from build123d import *

# Parameters (mm, degrees)
CYLINDER011_R     = 2.2
CYLINDER011_DEPTH = 10
CYLINDER012_R     = 2.2
CYLINDER012_DEPTH = 10
PAD015_DEPTH      = 6
CYLINDER013_R     = 4.5
CYLINDER013_DEPTH = 8


with BuildPart() as obj1:
    # Cylinder011 → Cylinder011 (new body)
    with BuildSketch(Plane(origin=(5, 0, -2), x_dir=(1, 0, 0), z_dir=(0, 0, 1))):
        Circle(CYLINDER011_R)
    extrude(amount=CYLINDER011_DEPTH)


with BuildPart() as double_hole_fusion:
    # Cylinder012 → Cylinder012 (new body)
    with BuildSketch(Plane(origin=(-5, 0, -2), x_dir=(1, 0, 0), z_dir=(0, 0, 1))):
        Circle(CYLINDER012_R)
    extrude(amount=CYLINDER012_DEPTH)

    # Fusion010: union obj1
    add(obj1.part)


with BuildPart() as body016:
    # Sketch016 → Pad015 (new body)
    with BuildSketch(Plane.XY):
        with BuildLine():
            Line((-5, 8), (5, 8))
            ThreePointArc((5, -8), (13, 0), (5, 8))
            Line((-5, -8), (5, -8))
            ThreePointArc((-5, 8), (-13, 0), (-5, -8))
        make_face()
    extrude(amount=PAD015_DEPTH)


with BuildPart() as simple_idle_linkage_cut:
    # Cylinder013 → Cylinder013 (new body)
    with BuildSketch(Plane(origin=(5, 0, 0), x_dir=(1, 0, 0), z_dir=(0, 0, 1))):
        Circle(CYLINDER013_R)
    extrude(amount=CYLINDER013_DEPTH)

    # Fusion011: union Body016
    add(body016.part)

    # Cut004: cut double hole fusion
    add(double_hole_fusion.part, mode=Mode.SUBTRACT)


solid = simple_idle_linkage_cut.part
Geometry: final body of the model. Coordinates: model frame, mm. Round coordinates to 2 decimals unless told otherwise and drop trailing zeros. Order: outer loops, then holes, each group sorted by start corner. A loop starts at its lowest first (then second) coordinate and runs counter-clockwise, first axis right, second up. Notation, with made-up numbers: (14, 54) -> (30, 54) arc R23 ccw to (30, 68) -> close; hole circle Ø7 at (25, -13.5). An arc over 180 degrees is marked (long way). Put each result on its own line as item: value. Start each with the question number.
Q1. Line query: probe 1 along X at (y, z) = (0, 5.75); probe 2 along X at (y, z) = (1, 5.75); probe 3 along Y at (x, z) = (-5, 3.9). Output: solid intervals per line, ascending.
Q2. Section A-A on y = 0. Return the cut outline in (x, z), and give its area (3 significant figures).
Q3. Section D-D on x = -10.5. Return the cut outline in (y, z).
Q4. Pull-direction query (Y, two-part tool) for faces 1 (the cylindrical face through (7.1, 0.66, 3.94)), 2 (the flat face through (3.9, 2.1, 8)), 3 (the cylindrical face through (9.292, 1.352, 6.986)); classes: +Y half, -Y half, draft (parallel to the pull), parting line (faces both ways), or undercut.
Q5. First-contact query: pin 1 (1.5 mm diameter, centred on x = -8.5, y = -3.5, fed in from +Z). Flat tip, straight axial feed; report the tip coordinate or a pass-through.
Q6. Section B-B on z = 3.5. Return the cut outline in (x, y).
Q7. Section C-C on y = -3.75. Return the cut outline in (x, z).
Ans:
1. probe 1: x = -13 to -7.2, -2.8 to 2.8, 7.2 to 13
1. probe 2: x = -12.94 to -6.96, -3.04 to 3.04, 6.96 to 12.94
1. probe 3: y = -8 to -2.2, 2.2 to 8
2. outline: (-13, 0) -> (-7.2, 0) -> (-7.2, 6) -> (-13, 6) -> close; (-2.8, 0) -> (2.8, 0) -> (2.8, 8) -> (0.5, 8) -> (0.5, 6) -> (-2.8, 6) -> close; (7.2, 0) -> (13, 0) -> (13, 6) -> (9.5, 6) -> (9.5, 8) -> (7.2, 8) -> close
2. area: 112 mm2
3. outline: (-5.81, 0) -> (5.81, 0) -> (5.81, 6) -> (-5.81, 6) -> close
4. face 1: undercut
4. face 2: draft
4. face 3: parting line
5. pin 1: stops at z = 6
6. outline: (-5, -8) -> (5, -8) arc R8 ccw to (5, 8) -> (-5, 8) arc R8 ccw to start; hole circle Ø4.4 at (-5, 0); hole circle Ø4.4 at (5, 0)
7. outline: (-12.07, 0) -> (12.07, 0) -> (12.07, 6) -> (7.49, 6) -> (7.49, 8) -> (2.51, 8) -> (2.51, 6) -> (-12.07, 6) -> close
